Design review of the part built by this model. Coordinates are the model's own, in mm. Face numbers are marked on the shaded views. Coordinates: 2 decimals unless noted, no trailing zeros. Loops run counter-clockwise (first coordinate to the right, second up) from the corner with the lowest first, then second, coordinate; pieces in that order, holes last. Notation, with made-up numbers: (68, 19.5) - (77, 19.5) arc R31 ccw to (77, 45.5) - close; hole circle Ø2 at (15.5, -38.5). An arc over 180 degrees is marked (long way). Return JSON: item names as keys, results as strings. Group by question number.
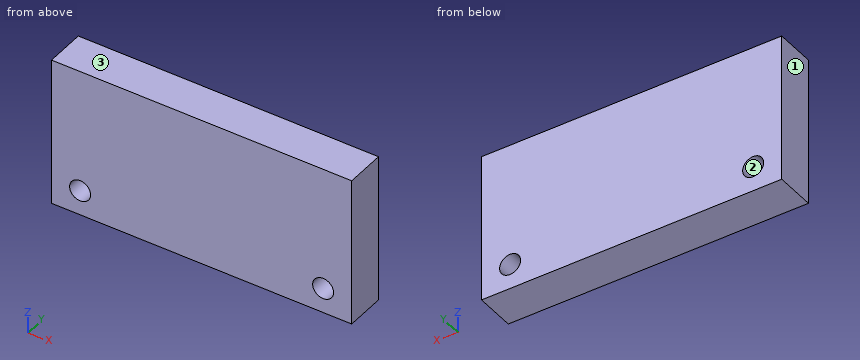
from build123d import *

# Parameters (mm, degrees)
SKETCH1_W           = 30
SKETCH1_H           = 5
SKETCH1_R           = 1.05
SKETCH1_H_2         = 9.890975922
BOSS_EXTRUDE1_DEPTH = 4


with BuildPart() as part:
    # Sketch1 → Boss-Extrude1 (new body)
    # profile 1 of 2: a face of its own
    with BuildSketch(Plane(origin=(0, 0, 0), x_dir=(1, 0, 0), z_dir=(0, 1, 0))):
        Rectangle(SKETCH1_W, SKETCH1_H)
        with Locations(Location((12.1449485, 0, 0), (0, 0, 270))):
            Circle(SKETCH1_R, mode=Mode.SUBTRACT)
        with Locations(Location((-12.1449485, 0, 0), (0, 0, 270))):
            Circle(SKETCH1_R, mode=Mode.SUBTRACT)
    # profile 2 of 2: a face of its own
    with BuildSketch(Plane(origin=(0, 0, 0), x_dir=(1, 0, 0), z_dir=(0, 1, 0))):
        with Locations((0, -7.445487961)):
            Rectangle(SKETCH1_W, SKETCH1_H_2)
    extrude(amount=BOSS_EXTRUDE1_DEPTH)


solid = part.part
Item 1: To check wall thickness, follow line 1 (X direction, y = 1.55, z = 0); line 2 (X direction, y = 3.1, z = -0.75); line 3 (Z direction, x = -12, y = 1.45). State the ranges of each line that lie inside material, in increasing order. Write a range as from..to.
Item 2: Add section A-A (z = 0). State the section outline as (x, y) points, then the cut area to 3 significant figures.
Item 3: Add section B-B (y = 2.8). State the section outline as (x, z) points.
Item 4: Draft analysis for pull direction Z (two halves, no side actions). For the marked faces 1, 2 and 3, state which applies: pulls with the +Z half, pulls with the -Z half, needs draft (parallel to the pull), parting line crosses it, or undercut.
Item 5: For P1, Ø1.9, axis at x = -12.14, z = 0, coming from the -Y side, flat-tipped, find the tip position at first contact; note if it passes through.
Answers below:
{
 "1": {"line 1": "x = -15..-13.19, -11.09..11.09, 13.19..15", "line 2": "x = -15..-12.88, -11.41..11.41, 12.88..15", "line 3": "z = -2.5..-1.04, 1.04..12.39"},
 "2": {"outline": "(-15, 0) - (-13.19, 0) - (-13.19, 4) - (-15, 4) - close; (-11.09, 0) - (11.09, 0) - (11.09, 4) - (-11.09, 4) - close; (13.19, 0) - (15, 0) - (15, 4) - (13.19, 4) - close", "area": "103 mm^2"},
 "3": {"outline": "(-15, -2.5) - (15, -2.5) - (15, 12.39) - (-15, 12.39) - close; hole circle Ø2.1 at (-12.14, 0); hole circle Ø2.1 at (12.14, 0)"},
 "4": {"face 1": "needs draft", "face 2": "undercut", "face 3": "pulls with the +Z half"},
 "5": {"P1": "passes through"}
}
